Can you work these out from the model? Positions are in its coordinate system, mm. A direction names the side the tool comes from. Coordinates: 2 decimals unless noted, no trailing zeros. Order: outer loops, then holes, each group sorted by start corner. A loop starts at its lowest first (then second) coordinate and runs counter-clockwise, first axis right, second up. Notation, with made-up numbers: (6, 2.25) -> (11, 2.25) arc R26 ccw to (11, 21.25) -> close; hole circle Ø9 at (60.5, 14). An arc over 180 degrees is marked (long way). Answer as a JSON object with one key per item and string values. Group by question number.
(1) I want a section at D-D, the plane z = -0.75. List the corners of the cut face in (x, y) for me (3 decimals), plus the area to 3 significant figures.
(2) Which directions (+Z, -Z, +X, -X, +Y, -Y) give clear straight access to the entire face, cutting with the end or side of a thin tool? Please do faces 1 (the cylindrical face through (-1.587, -2.837, 1.204)), 2 (the flat face through (-2, 5, 4.5)).
(3) For pin 1 (5 mm diameter, centred on x = 3.5, y = -0.5, fed in from +Z); pin 2 (2.5 mm diameter, centred on x = 4.25, y = 0, fed in from +Z); pin 3 (4 mm diameter, centred on y = -4, z = 6, fed in from -X); pin 4 (1.5 mm diameter, centred on x = 5.5, z = 5, fed in from +Y), each with a flat end and sliding along its axis, tell me the tip position at first contact or that it passes through.
(4) I want a section at B-B, the plane x = 4.25. List the corners of the cut face in (y, z) for me.
(5) If we mould it in two halves opening along Y, with no side actions, what happens to faces 3 (the cylindrical face through (3.25, 0.04, 1.2)), 4 (the cylindrical face through (-2.17, -9.76, 2.93)), 5 (the flat face through (0, 0, 8))? For each: pulls with the +Y half, pulls with the -Y half, needs draft (parallel to the pull), parting line crosses it, or undercut.
(6) I want a section at C-C, the plane y = 8. List the corners of the cut face in (x, z) for me.
(7) I need wall thicknesses on line 1 (Y direction, x = -0.5, z = 5.75); line 2 (Z direction, x = 5, y = -2); line 3 (Y direction, x = 0.25, z = 3.5). Which ranges of each line are inside material? Lowest first, please.
(8) I want a section at A-A, the plane y = 0. List the corners of the cut face in (x, z) for me.
from build123d import *

# Parameters (mm, degrees)
CYLINDER157_R     = 2.25
CYLINDER157_DEPTH = 7
CYLINDER156_R     = 1
CYLINDER156_DEPTH = 14
CYLINDER147_R     = 1
CYLINDER147_DEPTH = 1
ARRAY_COUNT       = 3
CYLINDER153_R     = 10
CYLINDER153_DEPTH = 10


with BuildPart() as sealsubtraction:
    # Cylinder157 → Cylinder157 (new body)
    with BuildSketch(Plane.XY.offset(4.5)):
        Circle(CYLINDER157_R)
    extrude(amount=CYLINDER157_DEPTH)


with BuildPart() as bottomwireoutlet:
    # Cylinder156 → Cylinder156 (new body)
    with BuildSketch(Plane.XY.offset(-7)):
        Circle(CYLINDER156_R)
    extrude(amount=CYLINDER156_DEPTH)


with BuildPart() as sealarray:
    # Cylinder147 → Cylinder147 (new body)
    with BuildSketch(Plane.XY.offset(4.5)):
        Circle(CYLINDER147_R)
    extrude(amount=CYLINDER147_DEPTH)

    # Fusion: union SealSubtraction, BottomWireOutlet
    add(sealsubtraction.part)
    add(bottomwireoutlet.part)


with BuildPart() as sealarray_1:
    # Fusion placement: moved
    add(sealarray.part.moved(Location((4.25, 0, 0))))

    # Array: SealArray ×3 about axis
    array_axis = Axis((0, 0, 0), (0, 0, 1))


with BuildPart() as sealarray_2:
    add(sealarray_1.part)
    for i in range(1, ARRAY_COUNT):
        add(sealarray_1.part.rotate(array_axis, i * 360 / ARRAY_COUNT))


with BuildPart() as cut:
    # Cylinder153 → Cylinder153 (new body)
    with BuildSketch(Plane.XY.offset(-2)):
        Circle(CYLINDER153_R)
    extrude(amount=CYLINDER153_DEPTH)

    # Cut: cut SealArray
    add(sealarray_2.part, mode=Mode.SUBTRACT)


solid = cut.part
Computed values:
{
 "1": {"outline": "circle Ø20 at (0, 0); hole circle Ø2 at (-2.125, -3.681); hole circle Ø2 at (-2.125, 3.681); hole circle Ø2 at (4.25, 0)", "area": "305 mm2"},
 "2": {"face 1": "+Z, -Z", "face 2": "+Z"},
 "3": {"pin 1": "stops at z = 8", "pin 2": "stops at z = 4.5", "pin 3": "stops at x = -9.8", "pin 4": "stops at y = 8.8"},
 "4": {"outline": "(-9.05, -2) -> (-1, -2) -> (-1, 4.5) -> (-2.25, 4.5) -> (-2.25, 8) -> (-9.05, 8) -> close; (1, -2) -> (9.05, -2) -> (9.05, 8) -> (2.25, 8) -> (2.25, 4.5) -> (1, 4.5) -> close"},
 "5": {"face 3": "undercut", "face 4": "parting line crosses it", "face 5": "needs draft"},
 "6": {"outline": "(-6, -2) -> (6, -2) -> (6, 8) -> (-6, 8) -> close"},
 "7": {"line 1": "y = -9.99 to -5.24, -2.12 to 2.12, 5.24 to 9.99", "line 2": "z = -2 to 4.5", "line 3": "y = -10 to 10"},
 "8": {"outline": "(-10, -2) -> (3.25, -2) -> (3.25, 4.5) -> (2, 4.5) -> (2, 8) -> (-10, 8) -> close; (5.25, -2) -> (10, -2) -> (10, 8) -> (6.5, 8) -> (6.5, 4.5) -> (5.25, 4.5) -> close"}
}
